from build123d import *

# Parameters (mm, degrees)
F0_W     = 53.975
F0_H     = 19.05
F1_DEPTH = 19.05
F2_W     = 60.325
F2_H     = 19.05
F3_DEPTH = 19.05
F4_W     = 30.1625
F4_H     = 19.05
F5_DEPTH = 19.05


# Not quite as in the source:
# - a length typed as a fraction of an inch, garbled in the dataset ("3 / 203.2 mm" for 3/8 in), is restored


with BuildPart() as f1:
    # F0 (on Top) → F1 (new body)
    with BuildSketch(Plane.XY):
        Polygon((53.975, -60.325), (53.975, 60.325), (-53.975, 60.325), (-53.975, -60.325), (-26.9875, -60.325), (-26.9875, -41.275), (26.9875, -41.275), (26.9875, -60.325), align=None)
        with Locations((0, -69.85)):
            Rectangle(F0_W, F0_H)
        with Locations((0, -50.8)):
            Rectangle(F0_W, F0_H)
    extrude(amount=F1_DEPTH)

    # F2 (on face) → F3 (cut)
    with BuildSketch(Plane.YZ.offset(53.975)):
        with Locations((0, 9.525)):
            Rectangle(F2_W, F2_H)
    extrude(amount=-F3_DEPTH, mode=Mode.SUBTRACT)

    # F4 (on face) → F5 (cut)
    with BuildSketch(Plane(origin=(-53.975, 0, 0), x_dir=(0, -1, 0), z_dir=(-1, 0, 0))):
        with Locations((-45.24375, 9.525)):
            Rectangle(F4_W, F4_H)
        with Locations((45.24375, 9.525)):
            Rectangle(F4_W, F4_H)
    extrude(amount=-F5_DEPTH, mode=Mode.SUBTRACT)


solid = f1.part
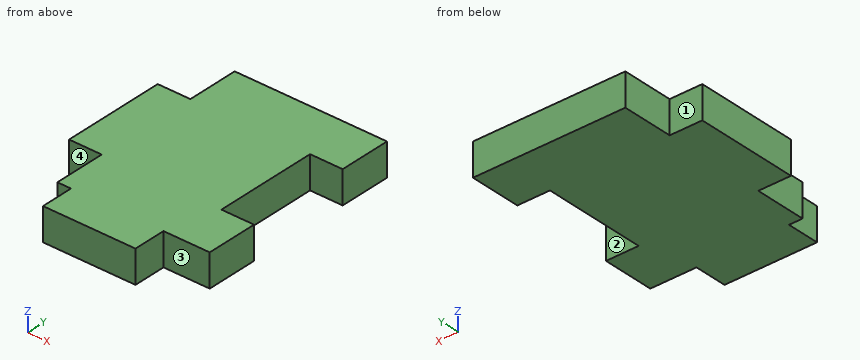
Model file for the job. Use its own axes, mm. Face numbers are marked on the shaded views. A direction names the side the tool comes from. Coordinates: 2 decimals unless noted, no trailing zeros. Order: outer loops, then holes, each group sorted by start corner. A loop starts at its lowest first (then second) coordinate and runs counter-clockwise, first axis right, second up. Notation, with made-up numbers: (-38, -1) -> (1, -1) arc R17 cw to (1, 18) -> close; hole circle Ø8 at (46, -35). An arc over 180 degrees is marked (long way). Return JSON: item names as keys, results as strings. Group by question number.
Item 1: Flat gauge pins, fed straight in: P1, Ø9.5, axis at y = 14.5, z = 9.5, coming from the +X side (3 decimals); P2, Ø6, axis at x = -36, z = 3.5, coming from the -Y side (3 decimals); P3, Ø5.5, axis at y = -65.5, z = 12, coming from the -X side; P4, Ø12, axis at x = -28, y = -63.5, coming from the +Z side. Where does each tip first touch, or does it go through?
Item 2: Wall check: line 1 along Y through (x, z) = (42, 1) (1 decimal); line 2 along Y through (x, z) = (-37, 6.25); line 3 along X through (y, z) = (-61, 10.5). Give the ranges that are in metal, low to high. Write a range as [from, to].
Item 3: Tool access for the marked faces 1, 2, 3 and 4: list every direction of +Z, -Z, +X, -X, +Y, -Y with a clear straight run to the whole face (end or side of a thin tool).
Item 4: Saw through at B-B on x = -38. Write the cut outline in (y, z).
Item 5: Saw through at A-A on z = 4.5. Write the cut outline in (x, y) (1 decimal), then the cut area to 3 significant figures.
Item 6: Saw through at C-C on y = 35. Write the cut outline in (x, z) (3 decimals), then the cut area to 3 significant figures.
Values found:
{
 "1": {"P1": "stops at x = 34.925", "P2": "stops at y = -60.325", "P3": "stops at x = -26.99", "P4": "stops at z = 19.05"},
 "2": {"line 1": "y = [-60.3, -30.2], [30.2, 60.3]", "line 2": "y = [-30.16, 30.16]", "line 3": "x = [-26.99, 26.99]"},
 "3": {"face 1": "+Z, -Z, -X, +Y", "face 2": "+Z, -Z, +X", "face 3": "+Z, -Z, +X, -Y", "face 4": "+Z, -Z, -X, -Y"},
 "4": {"outline": "(-30.16, 0) -> (30.16, 0) -> (30.16, 19.05) -> (-30.16, 19.05) -> close"},
 "5": {"outline": "(-54, -30.2) -> (-34.9, -30.2) -> (-34.9, -60.3) -> (-27, -60.3) -> (-27, -79.4) -> (27, -79.4) -> (27, -60.3) -> (54, -60.3) -> (54, -30.2) -> (34.9, -30.2) -> (34.9, 30.2) -> (54, 30.2) -> (54, 60.3) -> (-34.9, 60.3) -> (-34.9, 30.2) -> (-54, 30.2) -> close", "area": "11,800 mm2"},
 "6": {"outline": "(-34.925, 0) -> (53.975, 0) -> (53.975, 19.05) -> (-34.925, 19.05) -> close", "area": "1,690 mm2"}
}
